Geometry: final body of the model. Coordinates: model frame, mm. Coordinates: 2 decimals unless noted, no trailing zeros. Write each loop counter-clockwise with the first axis right and the second up, starting at its lowest first coordinate (ties: lowest second). Pieces come first, ordered by that corner, then holes. Notation, with made-up numbers: (66, 2.5) -> (102, 2.5) arc R30 ccw to (102, 41.5) -> close; hole circle Ø1 at (28.25, 64). An arc over 180 degrees is marked (long way). One line per item, written item: value.
```python
from build123d import *

# Parameters (mm, degrees)
F3_DEPTH      = 210
F3_DEPTH_BACK = 25
F5_DEPTH      = 210
F5_DEPTH_BACK = 25


with BuildPart() as f1:
    # F0 (on Front) → F1 (revolve)
    with BuildSketch(Plane.XZ):
        with BuildLine():
            Line((6, 40), (0, 40))
            Line((0, 40), (0, -40))
            Line((0, -40), (6, -40))
            Line((6, -40), (6, -35))
            ThreePointArc((6, -35), (7.121945325, -28.3955279025), (10.3619051686, -22.5320414644))
            ThreePointArc((10.3619051686, -22.5320414644), (16.1478700246, -11.9337677658), (17.9879737223, 0))
            ThreePointArc((17.9879737223, 0), (16.1478700246, 11.9337677658), (10.3619051686, 22.5320414644))
            ThreePointArc((10.3619051686, 22.5320414644), (7.121945325, 28.3955279025), (6, 35))
            Line((6, 35), (6, 40))
        make_face()
    revolve(axis=Axis((0, 0, 0), (0, 0, -1)))

    # F2 (on face) → F3 (join, two sides)
    with BuildSketch(Plane.XY.offset(40)) as f3_sk:
        with BuildLine():
            Line((6, 0), (6, 6))
            Line((6, 6), (0, 6))
            ThreePointArc((0, 6), (4.2426406871, 4.2426406871), (6, 0))
        make_face()
        with BuildLine():
            ThreePointArc((-6, 0), (-4.2426406871, 4.2426406871), (0, 6))
            Line((0, 6), (-6, 6))
            Line((-6, 6), (-6, 0))
        make_face()
        with BuildLine():
            ThreePointArc((0, -6), (-4.2426406871, -4.2426406871), (-6, 0))
            Line((-6, 0), (-6, -6))
            Line((-6, -6), (0, -6))
        make_face()
        with BuildLine():
            Line((6, -6), (6, 0))
            ThreePointArc((6, 0), (4.2426406871, -4.2426406871), (0, -6))
            Line((0, -6), (6, -6))
        make_face()
        with BuildLine():
            ThreePointArc((6, 0), (4.2426406871, 4.2426406871), (0, 6))
            ThreePointArc((0, 6), (-4.2426406871, 4.2426406871), (-6, 0))
            ThreePointArc((-6, 0), (-4.2426406871, -4.2426406871), (0, -6))
            ThreePointArc((0, -6), (4.2426406871, -4.2426406871), (6, 0))
        make_face()
    extrude(amount=F3_DEPTH)
    extrude(f3_sk.sketch, amount=-F3_DEPTH_BACK)

    # F4 (on face) → F5 (join, two sides)
    with BuildSketch(Plane(origin=(0, 0, -40), x_dir=(1, 0, 0), z_dir=(0, 0, -1))) as f5_sk:
        with BuildLine():
            Line((6, 0), (6, 6))
            Line((6, 6), (0, 6))
            ThreePointArc((0, 6), (4.2426406871, 4.2426406871), (6, 0))
        make_face()
        with BuildLine():
            ThreePointArc((-6, 0), (-4.2426406871, 4.2426406871), (0, 6))
            Line((0, 6), (-6, 6))
            Line((-6, 6), (-6, 0))
        make_face()
        with BuildLine():
            ThreePointArc((6, 0), (4.2426406871, 4.2426406871), (0, 6))
            ThreePointArc((0, 6), (-4.2426406871, 4.2426406871), (-6, 0))
            ThreePointArc((-6, 0), (-4.2426406871, -4.2426406871), (0, -6))
            ThreePointArc((0, -6), (4.2426406871, -4.2426406871), (6, 0))
        make_face()
        with BuildLine():
            Line((6, -6), (6, 0))
            ThreePointArc((6, 0), (4.2426406871, -4.2426406871), (0, -6))
            Line((0, -6), (6, -6))
        make_face()
        with BuildLine():
            ThreePointArc((0, -6), (-4.2426406871, -4.2426406871), (-6, 0))
            Line((-6, 0), (-6, -6))
            Line((-6, -6), (0, -6))
        make_face()
    extrude(amount=F5_DEPTH)
    extrude(f5_sk.sketch, amount=-F5_DEPTH_BACK)


solid = f1.part
```
(1) Line query: line 1 (X direction, y = -5, z = 147); line 2 (Z direction, x = 8.5, y = -3). Output: solid intervals per line, ascending. Write a range as [from, to].
Responses:
line 1: x = [-6, 6]
line 2: z = [-24.44, 24.44]
(2) First-contact query: pin 1 (2 mm diameter, centred on x = -5.5, z = -151.5, fed in from +Y); pin 2 (5 mm diameter, centred on y = 8, z = -178, fed in from -X); pin 3 (2 mm diameter, centred on x = 3, y = -9.5, fed in from +Z); pin 4 (8 mm diameter, centred on x = 13, z = -119, fed in from -Y). Flat tips, straight axial feed; report the tip coordinate or a pass-through.
Responses:
pin 1: stops at y = 6
pin 2: stops at x = -6
pin 3: stops at z = 24.53
pin 4: passes through
(3) Section A-A (z = -86.5). Return the cut outline in (x, y), then the cut area to 3 significant figures.
Responses:
outline: (-6, -6) -> (6, -6) -> (6, 6) -> (-6, 6) -> close
area: 144 mm2
